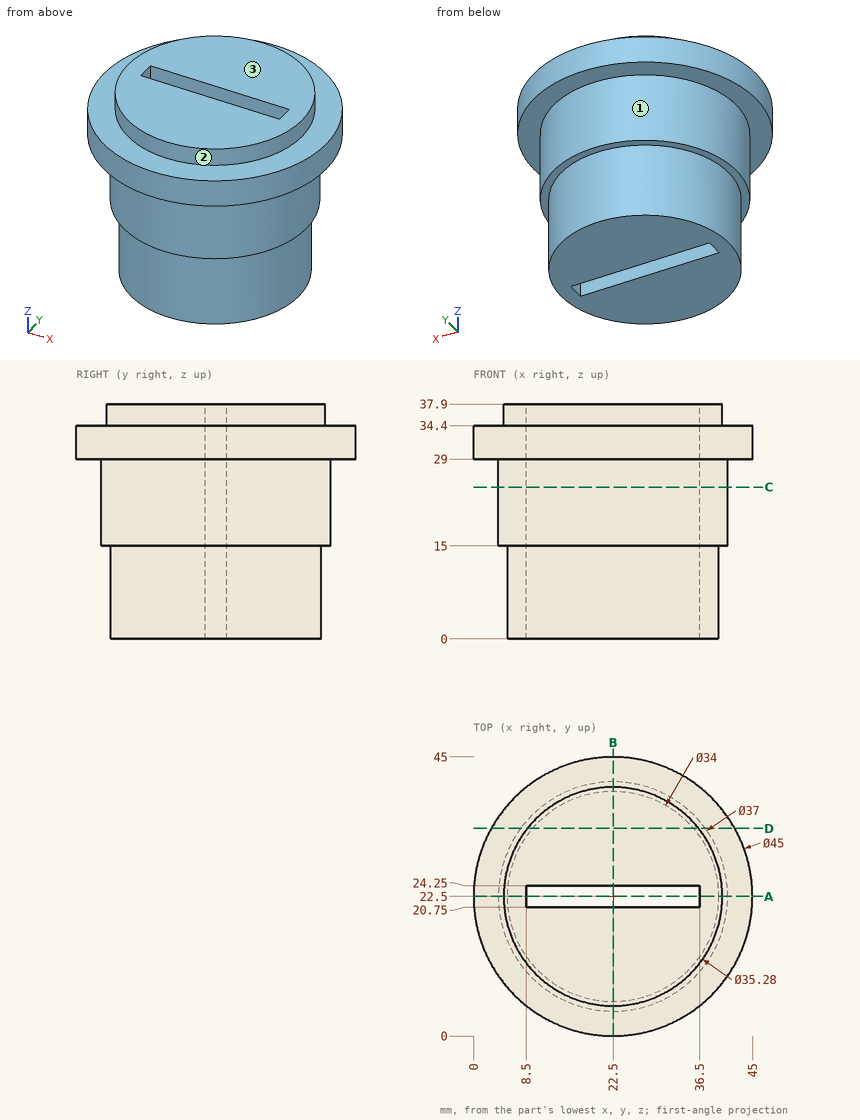
The drawing under review shows one solid part. Ordinate dimensions are in mm from its lowest x, y, z. A direction names the side the tool comes from. Coordinates: 2 decimals unless noted, no trailing zeros. Order: outer loops, then holes, each group sorted by start corner. A loop starts at its lowest first (then second) coordinate and runs counter-clockwise, first axis right, second up. Notation, with made-up numbers: M 55,66 L 90,66 A33 cw 90,102 Z; hole C -1.75,59 d8. An arc over 180 degrees is marked long. Use a Markdown table: item, result.
(1) Wall thickness on probe 1 along Y at (x, z) = (12, 16); probe 2 along Y at (x, z) = (17.5, 8.5); probe 3 along X at (y, z) = (21, 17): over which ranges is each line inside the solid? List them lowest first.
Worked answers:
| item | result |
|---|---|
| probe 1 | y = 7.27 to 20.75, 24.25 to 37.73 |
| probe 2 | y = 6.25 to 20.75, 24.25 to 38.75 |
| probe 3 | x = 4.06 to 8.5, 36.5 to 40.94 |
(2) For P1, Ø4, axis at y = 21.5, z = 27.5, coming from the -X side; P2, Ø2, axis at x = 21.5, z = 20, coming from the -Y side; P3, Ø3, axis at y = 21.5, z = 8, coming from the -X side; P4, Ø1, axis at y = 23, z = 22.5, coming from the +X side, all flat-tipped, find the tip position at first contact; note any pin that passes through.
Worked answers:
| item | result |
|---|---|
| P1 | stops at x = 0 |
| P2 | stops at y = 4 |
| P3 | stops at x = 5.5 |
| P4 | stops at x = 41 |
(3) Add section C-C (z = 24.5). Give the boundary of the cut face in (x, y), then the cut area to 3 significant figures.
Worked answers:
| item | result |
|---|---|
| outline | C 22.5,22.5 d37; hole M 8.5,20.75 L 36.5,20.75 L 36.5,24.25 L 8.5,24.25 Z |
| area | 977 mm2 |
(4) Add section A-A (y = 22.5). Give the boundary of the cut face in (x, z).
Worked answers:
| item | result |
|---|---|
| outline | M 0,29 L 4,29 L 4,15 L 5.5,15 L 5.5,0 L 8.5,0 L 8.5,37.9 L 4.86,37.9 L 4.86,34.4 L 0,34.4 Z; M 36.5,0 L 39.5,0 L 39.5,15 L 41,15 L 41,29 L 45,29 L 45,34.4 L 40.14,34.4 L 40.14,37.9 L 36.5,37.9 Z |
(5) For the marked faces 1, 2 and 3, list the 3-axis set-ups (+Z, -Z, +X, -X, +Y, -Y) from which the entire face can be reached by the end or side of a thin tool; tool diameter is ignored.
Worked answers:
| item | result |
|---|---|
| face 1 | -Z |
| face 2 | +Z |
| face 3 | +Z, +X, -X, +Y, -Y |
(6) Add section D-D (y = 33.5). Give the boundary of the cut face in (x, z), then the cut area to 3 significant figures.
Worked answers:
| item | result |
|---|---|
| outline | M 2.87,29 L 7.63,29 L 7.63,15 L 9.54,15 L 9.54,0 L 35.46,0 L 35.46,15 L 37.37,15 L 37.37,29 L 42.13,29 L 42.13,34.4 L 36.29,34.4 L 36.29,37.9 L 8.71,37.9 L 8.71,34.4 L 2.87,34.4 Z |
| area | 1,110 mm2 |
(7) Add section B-B (x = 22.5). Give the boundary of the cut face in (y, z).
Worked answers:
| item | result |
|---|---|
| outline | M 0,29 L 4,29 L 4,15 L 5.5,15 L 5.5,0 L 20.75,0 L 20.75,37.9 L 4.86,37.9 L 4.86,34.4 L 0,34.4 Z; M 24.25,0 L 39.5,0 L 39.5,15 L 41,15 L 41,29 L 45,29 L 45,34.4 L 40.14,34.4 L 40.14,37.9 L 24.25,37.9 Z |
